from build123d import *

# Parameters (mm, degrees)
SKETCH1_W               = 104.902
SKETCH1_H               = 47.752
EXTRUDE1_DEPTH          = 16.002
FILLET1_R               = 6.35
SKETCH2_W               = 104.902
SKETCH2_H               = 16.002
EXTRUDE2_DEPTH          = 69.85
CUT_EXTRUDE1_DEPTH      = 69.85
CUT_EXTRUDE3_DEPTH      = 32.75
CUT_EXTRUDE3_DEPTH_BACK = 17.002
SKETCH5_R               = 19.05
EXTRUDE3_DEPTH          = 19.05
SKETCH6_R               = 8.001
CUT_EXTRUDE4_DEPTH      = 36.052


with BuildPart() as part:
    # Sketch1 → Extrude1 (new body)
    with BuildSketch(Plane(origin=(0, 0, 0), x_dir=(1, 0, 0), z_dir=(0, 1, 0))):
        with Locations((-26.583821429, -19.496767857)):
            Rectangle(SKETCH1_W, SKETCH1_H)
    extrude(amount=EXTRUDE1_DEPTH)

    # Fillet1
    fillet1_edges = [part.edges().sort_by_distance(p)[0] for p in [
        (25.867178571, 8.001, 43.372767857),
        (-79.034821429, 8.001, 43.372767857),
    ]]
    fillet(fillet1_edges, radius=FILLET1_R)

    # Sketch2 → Extrude2 (add)
    with BuildSketch(Plane(origin=(0, 16.002, 0), x_dir=(-1, 0, 0), z_dir=(0, 1, 0))):
        with Locations((26.583821429, 3.621767857)):
            Rectangle(SKETCH2_W, SKETCH2_H)
    extrude(amount=EXTRUDE2_DEPTH)

    # Sketch3 → Cut-Extrude1 (cut)
    with BuildSketch(Plane.XY.offset(11.622767857)):
        with BuildLine():
            ThreePointArc((-59.984821429, 85.852), (-53.216510402, 84.609090325), (-47.331390899, 81.042547596))
            Line((-47.331390899, 81.042547596), (25.867178571, 16.002))
            Line((25.867178571, 16.002), (25.867178571, 85.852))
            Line((25.867178571, 85.852), (-59.984821429, 85.852))
        make_face()
    extrude(amount=-CUT_EXTRUDE1_DEPTH, mode=Mode.SUBTRACT)

    # Sketch4 → Cut-Extrude3 (cut, two sides)
    with BuildSketch(Plane.XY.offset(11.622767857)) as cut_extrude3_sk:
        with BuildLine():
            Line((198.747458809, 85.852), (-59.984821429, 85.852))
            ThreePointArc((-59.984821429, 85.852), (-73.45520561, 80.272384182), (-79.034821429, 66.802))
            Line((-79.034821429, 66.802), (-79.034821429, -191.930280237))
            Line((-79.034821429, -191.930280237), (-444.937521164, 173.972419498))
            Line((-444.937521164, 173.972419498), (-167.155240927, 451.754699735))
            Line((-167.155240927, 451.754699735), (198.747458809, 85.852))
        make_face()
    extrude(amount=CUT_EXTRUDE3_DEPTH, mode=Mode.SUBTRACT)
    extrude(cut_extrude3_sk.sketch, amount=-CUT_EXTRUDE3_DEPTH_BACK, mode=Mode.SUBTRACT)

    # Sketch5 → Extrude3 (add)
    with BuildSketch(Plane.XY.offset(11.622767857)):
        with Locations((-59.984821429, 66.802)):
            Circle(SKETCH5_R)
    extrude(amount=EXTRUDE3_DEPTH)

    # Sketch6 → Cut-Extrude4 (cut, through all)
    with BuildSketch(Plane.XY.offset(30.672767857)):
        with Locations((-59.984821429, 66.802)):
            Circle(SKETCH6_R)
    extrude(amount=-CUT_EXTRUDE4_DEPTH, mode=Mode.SUBTRACT)


solid = part.part
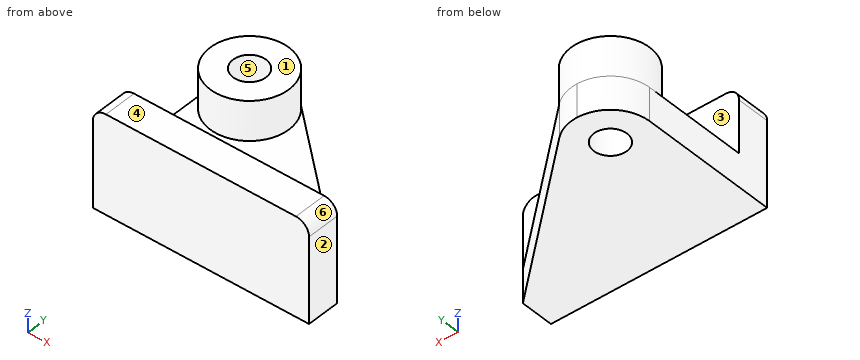
Design review of the part built by this model. Coordinates are the model's own, in mm. Face numbers are marked on the shaded views. A direction names the side the tool comes from. Round coordinates to 2 decimals unless told otherwise and drop trailing zeros. Loops run counter-clockwise (first coordinate to the right, second up) from the corner with the lowest first, then second, coordinate; pieces in that order, holes last. Notation, with made-up numbers: (66.5, -12.75) - (88.5, -12.75) arc R20 cw to (88.5, -5.75) - close; hole circle Ø9 at (68, -27). An arc over 180 degrees is marked (long way). One line per item, written item: value. Start each with the question number.
1) Insertion check: pin 1 Ø2 at (x, z) = (-23, 35) entering from +Y; pin 2 Ø4 at (x, z) = (-44.5, 22) entering from +Y; pin 3 Ø3 at (x, y) = (-30, 63) entering from +Z; pin 4 Ø5 at (x, y) = (4, 35.5) entering from -Z. Each pin has a flat end and moves straight along its axis. Give the tip position at first contact, or say it passes through.
2) Consider section D-D on x = -15.5. Give the boundary of the cut face in (y, z).
3) For the marked faces 1, 2 and 3, list the 3-axis set-ups (+Z, -Z, +X, -X, +Y, -Y) from which the entire face can be reached by the end or side of a thin tool; tool diameter is ignored.
4) To check wall thickness, follow L1, parallel to Z at x = -31, y = 44; L2, parallel to Y at x = 18.5, z = 15; L3, parallel to Z at x = -51.5, y = 63. State the ranges of each line that lie inside material, in increasing order. Write a range as from..to.
5) Consider section B-B on z = 9. Give the boundary of the cut face in (x, y), then the cut area to 3 significant figures.
6) Draft analysis for pull direction X (two halves, no side actions). For the marked faces 4, 5 and 6, state which applies: +X half, -X half, draft (parallel to the pull), parting line (faces both ways), or undercut.
7) Consider section C-C on y = 69. Give the boundary of the cut face in (x, z), then the cut area to 3 significant figures.
8) Consider section A-A on z = 27. Give the boundary of the cut face in (x, y), then the cut area to 3 significant figures.
Reported:
1. pin 1: stops at y = 16
1. pin 2: stops at y = 80.26
1. pin 3: stops at z = 11.62
1. pin 4: stops at z = -4.38
2. outline: (0, -4.38) - (52.76, -4.38) - (52.76, 11.62) - (16, 11.62) - (16, 43.37) - (0, 43.37) - close
3. face 1: +Z, +X, -X, +Y
3. face 2: +Z, -Z, +X, +Y, -Y
3. face 3: +Z, +X, -X
4. L1: z = -4.38..11.62
4. L2: y = 0..16
4. L3: z = -4.38..30.67
5. outline: (-79.03, 0) - (25.87, 0) - (25.87, 16) - (-47.33, 81.04) arc R19.05 ccw to (-79.03, 66.8) - close; hole circle Ø16 at (-59.98, 66.8)
5. area: 5,980 mm^2
6. face 4: draft
6. face 5: undercut
6. face 6: +X half
7. outline: (-78.91, -4.38) - (-67.68, -4.38) - (-67.68, 30.67) - (-78.91, 30.67) - close; (-52.29, -4.38) - (-33.78, -4.38) - (-33.78, 11.62) - (-41.06, 11.62) - (-41.06, 30.67) - (-52.29, 30.67) - close
7. area: 904 mm^2
8. outline: (-79.03, 0) - (25.87, 0) - (25.87, 16) - (-79.03, 16) - close; circle Ø38.1 at (-59.98, 66.8); hole circle Ø16 at (-59.98, 66.8)
8. area: 2,620 mm^2
